from build123d import *
from build123d import SkipClean  # not in build123d's __all__

# Parameters (mm, degrees)
F0_R     = 4.9113239183
F1_DEPTH = 5.08
F2_DEPTH = 2.54
F4_DEPTH = 2.54
F5_DEPTH = 5.08


# Not quite as in the source:
# - a feature names something its author has since deleted; it is built from what else it names


with BuildPart() as f1:
    # F0 (on Front) → F1 (new body)
    with BuildSketch(Plane.XZ):
        Polygon((11.684, -8.5716721153), (-11.684, -8.5716721153), (-12.7, -10.3314357358), (-13.716, -12.0911993563), (-2.032, -32.3284809919), (0, -32.3284809919), (2.032, -32.3284809919), (13.716, -12.0911993563), (12.7, -10.3314357358), align=None)
        with Locations((0, -18.7316721153)):
            Circle(F0_R, mode=Mode.SUBTRACT)
        with BuildLine():
            ThreePointArc((-11.4414768653, -3.5657760746), (-10.5023439874, -4.227888231), (-9.525, -4.8321744218))
            Line((-9.525, -4.8321744218), (0, 11.6656095203))
            Line((0, 11.6656095203), (0, 16.7456095203))
            Line((0, 16.7456095203), (-11.4414768653, -3.5657760746))
        make_face()
        with BuildLine():
            Line((9.525, -4.8321744218), (11.684, -8.5716721153))
            Line((11.684, -8.5716721153), (12.7, -10.3314357358))
            Line((12.7, -10.3314357358), (13.716, -12.0911993563))
            Line((13.716, -12.0911993563), (15.875, -15.8306970498))
            ThreePointArc((15.875, -15.8306970498), (16.8251832643, -15.3174546282), (17.8029235649, -14.8588808351))
            Line((17.8029235649, -14.8588808351), (11.4414768653, -3.5657760746))
            ThreePointArc((11.4414768653, -3.5657760746), (10.5023439874, -4.227888231), (9.525, -4.8321744218))
        make_face()
        with BuildLine():
            Line((0, 16.7456095203), (0, 11.6656095203))
            Line((0, 11.6656095203), (9.525, -4.8321744218))
            ThreePointArc((9.525, -4.8321744218), (10.5023439874, -4.227888231), (11.4414768653, -3.5657760746))
            Line((11.4414768653, -3.5657760746), (0, 16.7456095203))
        make_face()
        with BuildLine():
            Line((-25.4, -32.3284809919), (-15.875, -15.8306970498))
            ThreePointArc((-15.875, -15.8306970498), (-16.8251832643, -15.3174546282), (-17.8029235649, -14.8588808351))
            Line((-17.8029235649, -14.8588808351), (-29.4044214139, -35.4543423357))
            Line((-29.4044214139, -35.4543423357), (-25.4, -32.3284809919))
        make_face()
        with BuildLine():
            Line((0, -32.3284809919), (-2.032, -32.3284809919))
            Line((-2.032, -32.3284809919), (-6.35, -32.3284809919))
            ThreePointArc((-6.35, -32.3284809919), (-6.4146614456, -33.8967347902), (-6.6082068216, -35.4543423357))
            Line((-6.6082068216, -35.4543423357), (6.6082068216, -35.4543423357))
            ThreePointArc((6.6082068216, -35.4543423357), (6.4146614456, -33.8967347902), (6.35, -32.3284809919))
            Line((6.35, -32.3284809919), (2.032, -32.3284809919))
            Line((2.032, -32.3284809919), (0, -32.3284809919))
        make_face()
        with BuildLine():
            Line((-6.35, -32.3284809919), (-25.4, -32.3284809919))
            Line((-25.4, -32.3284809919), (-29.4044214139, -35.4543423357))
            Line((-29.4044214139, -35.4543423357), (-6.6082068216, -35.4543423357))
            ThreePointArc((-6.6082068216, -35.4543423357), (-6.4146614456, -33.8967347902), (-6.35, -32.3284809919))
        make_face()
        with BuildLine():
            Line((29.4044214139, -35.4543423357), (17.8029235649, -14.8588808351))
            ThreePointArc((17.8029235649, -14.8588808351), (16.8251832643, -15.3174546282), (15.875, -15.8306970498))
            Line((15.875, -15.8306970498), (25.4, -32.3284809919))
            Line((25.4, -32.3284809919), (29.4044214139, -35.4543423357))
        make_face()
        with BuildLine():
            ThreePointArc((6.35, -32.3284809919), (6.4146614456, -33.8967347902), (6.6082068216, -35.4543423357))
            Line((6.6082068216, -35.4543423357), (29.4044214139, -35.4543423357))
            Line((29.4044214139, -35.4543423357), (25.4, -32.3284809919))
            Line((25.4, -32.3284809919), (6.35, -32.3284809919))
        make_face()
    extrude(amount=F1_DEPTH)

    # F0 (on Front) → F2 (join)
    with BuildSketch(Plane.XZ):
        with BuildLine():
            ThreePointArc((19.05, 11.6656095203), (-8.5130008139, 28.7076550883), (-11.4414768653, -3.5657760746))
            Line((-11.4414768653, -3.5657760746), (0, 16.7456095203))
            Line((0, 16.7456095203), (11.4414768653, -3.5657760746))
            ThreePointArc((11.4414768653, -3.5657760746), (17.042045568, 3.1526087064), (19.05, 11.6656095203))
        make_face()
        with BuildLine():
            Line((0, 11.6656095203), (-9.525, -4.8321744218))
            ThreePointArc((-9.525, -4.8321744218), (0, -7.3843904797), (9.525, -4.8321744218))
            Line((9.525, -4.8321744218), (0, 11.6656095203))
        make_face()
        with BuildLine():
            Line((-29.4044214139, -35.4543423357), (-17.8029235649, -14.8588808351))
            ThreePointArc((-17.8029235649, -14.8588808351), (-42.1372748222, -41.4260703169), (-6.6082068216, -35.4543423357))
            Line((-6.6082068216, -35.4543423357), (-29.4044214139, -35.4543423357))
        make_face()
        with BuildLine():
            ThreePointArc((-6.35, -32.3284809919), (-8.9022160579, -22.8034809919), (-15.875, -15.8306970498))
            Line((-15.875, -15.8306970498), (-25.4, -32.3284809919))
            Line((-25.4, -32.3284809919), (-6.35, -32.3284809919))
        make_face()
        with BuildLine():
            ThreePointArc((44.45, -32.3284809919), (35.8445726076, -16.3969586841), (17.8029235649, -14.8588808351))
            Line((17.8029235649, -14.8588808351), (29.4044214139, -35.4543423357))
            Line((29.4044214139, -35.4543423357), (6.6082068216, -35.4543423357))
            ThreePointArc((6.6082068216, -35.4543423357), (26.9682537983, -51.3138195463), (44.45, -32.3284809919))
        make_face()
        with BuildLine():
            Line((25.4, -32.3284809919), (15.875, -15.8306970498))
            ThreePointArc((15.875, -15.8306970498), (8.9022160579, -22.8034809919), (6.35, -32.3284809919))
            Line((6.35, -32.3284809919), (25.4, -32.3284809919))
        make_face()
        with BuildLine():
            Line((-6.35, -32.3284809919), (-25.4, -32.3284809919))
            Line((-25.4, -32.3284809919), (-29.4044214139, -35.4543423357))
            Line((-29.4044214139, -35.4543423357), (-6.6082068216, -35.4543423357))
            ThreePointArc((-6.6082068216, -35.4543423357), (-6.4146614456, -33.8967347902), (-6.35, -32.3284809919))
        make_face()
        with BuildLine():
            Line((-25.4, -32.3284809919), (-15.875, -15.8306970498))
            ThreePointArc((-15.875, -15.8306970498), (-16.8251832643, -15.3174546282), (-17.8029235649, -14.8588808351))
            Line((-17.8029235649, -14.8588808351), (-29.4044214139, -35.4543423357))
            Line((-29.4044214139, -35.4543423357), (-25.4, -32.3284809919))
        make_face()
        with BuildLine():
            ThreePointArc((6.35, -32.3284809919), (6.4146614456, -33.8967347902), (6.6082068216, -35.4543423357))
            Line((6.6082068216, -35.4543423357), (29.4044214139, -35.4543423357))
            Line((29.4044214139, -35.4543423357), (25.4, -32.3284809919))
            Line((25.4, -32.3284809919), (6.35, -32.3284809919))
        make_face()
        with BuildLine():
            Line((29.4044214139, -35.4543423357), (17.8029235649, -14.8588808351))
            ThreePointArc((17.8029235649, -14.8588808351), (16.8251832643, -15.3174546282), (15.875, -15.8306970498))
            Line((15.875, -15.8306970498), (25.4, -32.3284809919))
            Line((25.4, -32.3284809919), (29.4044214139, -35.4543423357))
        make_face()
        with BuildLine():
            Line((0, 16.7456095203), (0, 11.6656095203))
            Line((0, 11.6656095203), (9.525, -4.8321744218))
            ThreePointArc((9.525, -4.8321744218), (10.5023439874, -4.227888231), (11.4414768653, -3.5657760746))
            Line((11.4414768653, -3.5657760746), (0, 16.7456095203))
        make_face()
        with BuildLine():
            ThreePointArc((-11.4414768653, -3.5657760746), (-10.5023439874, -4.227888231), (-9.525, -4.8321744218))
            Line((-9.525, -4.8321744218), (0, 11.6656095203))
            Line((0, 11.6656095203), (0, 16.7456095203))
            Line((0, 16.7456095203), (-11.4414768653, -3.5657760746))
        make_face()
    extrude(amount=-F2_DEPTH)

    # F3 (on face) → F4 (join)
    with BuildSketch(Plane.XZ.offset(5.08)):
        with BuildLine():
            ThreePointArc((11.4414768653, -3.5657760746), (17.042045568, 3.1526087064), (19.05, 11.6656095203))
            ThreePointArc((19.05, 11.6656095203), (-8.5130008139, 28.7076550883), (-11.4414768653, -3.5657760746))
            Line((-11.4414768653, -3.5657760746), (0, 16.7456095203))
            Line((0, 16.7456095203), (11.4414768653, -3.5657760746))
        make_face()
        with BuildLine():
            Line((0, 16.7456095203), (-11.4414768653, -3.5657760746))
            ThreePointArc((-11.4414768653, -3.5657760746), (-10.5023439874, -4.227888231), (-9.525, -4.8321744218))
            Line((-9.525, -4.8321744218), (0, 11.6656095203))
            Line((0, 11.6656095203), (9.525, -4.8321744218))
            ThreePointArc((9.525, -4.8321744218), (10.5023439874, -4.227888231), (11.4414768653, -3.5657760746))
            Line((11.4414768653, -3.5657760746), (0, 16.7456095203))
        make_face()
        with BuildLine():
            Line((0, 11.6656095203), (-9.525, -4.8321744218))
            ThreePointArc((-9.525, -4.8321744218), (0, -7.3843904797), (9.525, -4.8321744218))
            Line((9.525, -4.8321744218), (0, 11.6656095203))
        make_face()
        with BuildLine():
            Line((29.4044214139, -35.4543423357), (17.8029235649, -14.8588808351))
            ThreePointArc((17.8029235649, -14.8588808351), (16.8251832643, -15.3174546282), (15.875, -15.8306970498))
            Line((15.875, -15.8306970498), (25.4, -32.3284809919))
            Line((25.4, -32.3284809919), (6.35, -32.3284809919))
            ThreePointArc((6.35, -32.3284809919), (6.4146614456, -33.8967347902), (6.6082068216, -35.4543423357))
            Line((6.6082068216, -35.4543423357), (29.4044214139, -35.4543423357))
        make_face()
        with BuildLine():
            ThreePointArc((44.45, -32.3284809919), (35.8445726076, -16.3969586841), (17.8029235649, -14.8588808351))
            Line((17.8029235649, -14.8588808351), (29.4044214139, -35.4543423357))
            Line((29.4044214139, -35.4543423357), (6.6082068216, -35.4543423357))
            ThreePointArc((6.6082068216, -35.4543423357), (26.9682537983, -51.3138195463), (44.45, -32.3284809919))
        make_face()
        with BuildLine():
            Line((25.4, -32.3284809919), (15.875, -15.8306970498))
            ThreePointArc((15.875, -15.8306970498), (8.9022160579, -22.8034809919), (6.35, -32.3284809919))
            Line((6.35, -32.3284809919), (25.4, -32.3284809919))
        make_face()
        with BuildLine():
            Line((-29.4044214139, -35.4543423357), (-6.6082068216, -35.4543423357))
            ThreePointArc((-6.6082068216, -35.4543423357), (-6.4146614456, -33.8967347902), (-6.35, -32.3284809919))
            Line((-6.35, -32.3284809919), (-25.4, -32.3284809919))
            Line((-25.4, -32.3284809919), (-15.875, -15.8306970498))
            ThreePointArc((-15.875, -15.8306970498), (-16.8251832643, -15.3174546282), (-17.8029235649, -14.8588808351))
            Line((-17.8029235649, -14.8588808351), (-29.4044214139, -35.4543423357))
        make_face()
        with BuildLine():
            ThreePointArc((-17.8029235649, -14.8588808351), (-42.1372748222, -41.4260703169), (-6.6082068216, -35.4543423357))
            Line((-6.6082068216, -35.4543423357), (-29.4044214139, -35.4543423357))
            Line((-29.4044214139, -35.4543423357), (-17.8029235649, -14.8588808351))
        make_face()
        with BuildLine():
            Line((-25.4, -32.3284809919), (-6.35, -32.3284809919))
            ThreePointArc((-6.35, -32.3284809919), (-8.9022160579, -22.8034809919), (-15.875, -15.8306970498))
            Line((-15.875, -15.8306970498), (-25.4, -32.3284809919))
        make_face()
    with SkipClean():  # cleaning this boolean's faces spoils the solid; the shape is the same uncleaned
        extrude(amount=F4_DEPTH)

    # F0 (on Front) → F5 (join)
    with BuildSketch(Plane.XZ):
        Polygon((11.684, -8.5716721153), (-11.684, -8.5716721153), (-12.7, -10.3314357358), (-13.716, -12.0911993563), (-2.032, -32.3284809919), (0, -32.3284809919), (2.032, -32.3284809919), (13.716, -12.0911993563), (12.7, -10.3314357358), align=None)
        with Locations((0, -18.7316721153)):
            Circle(F0_R, mode=Mode.SUBTRACT)
        with BuildLine():
            Line((-12.7, -10.3314357358), (-11.684, -8.5716721153))
            Line((-11.684, -8.5716721153), (-9.525, -4.8321744218))
            ThreePointArc((-9.525, -4.8321744218), (-10.5023439874, -4.227888231), (-11.4414768653, -3.5657760746))
            Line((-11.4414768653, -3.5657760746), (-17.8029235649, -14.8588808351))
            ThreePointArc((-17.8029235649, -14.8588808351), (-16.8251832643, -15.3174546282), (-15.875, -15.8306970498))
            Line((-15.875, -15.8306970498), (-13.716, -12.0911993563))
            Line((-13.716, -12.0911993563), (-12.7, -10.3314357358))
        make_face()
    extrude(amount=F5_DEPTH)


solid = f1.part
Model file for the job. Use its own axes, mm. A direction names the side the tool comes from. Round coordinates to 2 decimals unless told otherwise and drop trailing zeros. Loops run counter-clockwise (first coordinate to the right, second up) from the corner with the lowest first, then second, coordinate; pieces in that order, holes last. Notation, with made-up numbers: M -27.5,32.5 L 29.5,32.5 A14 ccw 29.5,53.5 Z; hole C 20,-34.5 d7. An arc over 180 degrees is marked long. One line per question, with ' | ' between items.
1) Band-saw the part on B-B (z = -38.5). Give the cut face in (x, y).
Solved:
outline: M -43.42,-7.62 L -7.38,-7.62 L -7.38,-5.08 L -43.42,-5.08 Z; M -43.42,0 L -7.38,0 L -7.38,2.54 L -43.42,2.54 Z; M 7.38,-7.62 L 43.42,-7.62 L 43.42,-5.08 L 7.38,-5.08 Z; M 7.38,0 L 43.42,0 L 43.42,2.54 L 7.38,2.54 Z
2) Band-saw the part on A-A (x = -36). Give the cut face in (y, z), then the cut area to 3 significant figures.
Solved:
outline: M -7.62,-48.16 L -5.08,-48.16 L -5.08,-16.5 L -7.62,-16.5 Z; M 0,-48.16 L 2.54,-48.16 L 2.54,-16.5 L 0,-16.5 Z | area: 161 mm²
3) Drill centre lines: line 1 along X through (y, z) = (-0.5, -17.5); line 2 along Y through (x, z) = (-12, 19); line 3 along X through (y, z) = (-2.25, -29). Where is each one in solid material? Low to high.
Solved:
line 1: x = -19.29 to -16.84, -10.59 to -4.75, 4.75 to 10.59, 16.84 to 19.29 | line 2: y = -7.62 to -5.08, 0 to 2.54 | line 3: x = -25.77 to -23.48, -3.95 to 3.95, 23.48 to 25.77
4) Band-saw the part on C-C (y = 1.5). Give the cut face in (x, z) (3 decimals), then the cut area to 3 significant figures.
Solved:
outline: C -25.4,-32.328 d38.1; C 0,11.666 d38.1; C 25.4,-32.328 d38.1 | area: 3,420 mm²
5) Band-saw the part on D-D (z = 25.5). Give the cut face in (x, y), then the cut area to 3 significant figures.
Solved:
outline: M -13.1,-7.62 L 13.1,-7.62 L 13.1,-5.08 L -13.1,-5.08 Z; M -13.1,0 L 13.1,0 L 13.1,2.54 L -13.1,2.54 Z | area: 133 mm²
6) Flat gauge pins, fed straight in: pin 1 (1.5 mm diameter, centred on x = 13.5, y = -3, fed in from +Z); pin 2 (5 mm diameter, centred on x = -34.5, y = -3.5, fed in from -Z); pin 3 (4 mm diameter, centred on y = -5, z = 18.5, fed in from -X); pin 4 (9.5 mm diameter, centred on x = 8.5, z = -16.5, fed in from +Y). Where does each tip first touch, or does it go through?
Solved:
pin 1: stops at z = -5.89 | pin 2: stops at z = -49.98 | pin 3: stops at x = -18.43 | pin 4: stops at y = 2.54
7) Mould opens along Z. For faces 1 (the flat face through (-7.956, -2.504, -22.068)), 2 (the flat face through (0, -7.62, 12)), 3 (the flat face through (0, -3, -35.454)) say: +Z half, -Z half, draft (parallel to the pull), parting line (faces both ways), or undercut.
Solved:
face 1: undercut | face 2: draft | face 3: -Z half
8) 3-axis set-ups, long thin cutter, end or side, ignore diameter. For faces 4 (the flat face through (-4.2, -5.08, -15.7)), 5 (the flat face through (-14, 0, -26)), 6 (the flat face through (0, -5.08, 18)), 7 (the flat face through (-30, -5.08, -36)): which of +Z, -Z, +X, -X, +Y, -Y reach the whole face in a straight line?
Solved:
face 4: -Y | face 5: none | face 6: +Z | face 7: -X
